from build123d import *

# Parameters (mm, degrees)
F2_T     = 3.175
F3_R     = 6.35
F4_DEPTH = 64.008
F5_DEPTH = 104.14


# Not quite as in the source:
# - a shell that OpenCascade refuses in one call is made with other operations: the cavity is built on its own and cut out


with BuildPart() as f1:
    # F0 (on Top) → F1 (revolve)
    with BuildSketch(Plane.XY):
        Polygon((-37.0614958425, 0), (0, 0), (0, 59.2983933481), (-37.0614958425, 59.2983933481), (-37.0614958425, 54.4952234869), (-29.1296224819, 54.4952234869), (-29.1296224819, 50.8915618087), (-37.0614958425, 50.8915618087), (-37.0614958425, 46.1002111902), (-29.1296224819, 46.1002111902), (-29.1296224819, 42.483009196), (-37.0614958425, 42.483009196), (-37.0614958425, 37.6798393348), (-29.1296224819, 37.6798393348), (-29.1296224819, 31.75), (-37.0614958425, 31.75), align=None)
    revolve(axis=Axis((0, 29.649196674, 0), (0, 1, 0)))

    # F2: shell of thickness 3.175, made by hand


with BuildPart() as f2_core1:
    # F2_t2: copy of F1
    add(f1.part)

    # the walls: a layer under each face that stays
    f2_faces = [f2_core1.faces().sort_by_distance(p)[0] for p in [
        (29.1296224819, 34.7149196674, 0),
        (-24.707663895, 31.75, -24.707663895),
        (37.0614958425, 15.875, 0),
        (0, 59.2983933481, 0),
        (37.0614958425, 56.8968084175, 0),
        (24.707663895, 54.4952234869, -24.707663895),
        (29.1296224819, 52.6933926478, 0),
        (-24.707663895, 50.8915618087, -24.707663895),
        (37.0614958425, 48.4958864995, 0),
        (24.707663895, 46.1002111902, -24.707663895),
        (29.1296224819, 44.2916101931, 0),
        (-24.707663895, 42.483009196, -24.707663895),
        (37.0614958425, 40.0814242654, 0),
        (24.707663895, 37.6798393348, -24.707663895),
    ]]
    thicken(f2_faces, amount=-F2_T, mode=Mode.SUBTRACT)

    # F2_s3 → F2_t4 (revolve, cut)
    with BuildSketch(Plane.XY):
        Polygon((-29.1613724819, 37.6480893348), (-25.9546224819, 37.6798393348), (-25.9546224819, 40.8548393348), (-29.1296224819, 40.8548393348), align=None)
    revolve(axis=Axis((0, 37.6798393348, 0), (0, 1, 0)), mode=Mode.SUBTRACT)

    # F2_s5 → F2_t6 (revolve, cut)
    with BuildSketch(Plane.XY):
        Polygon((-29.1613724819, 31.78175), (-25.9546224819, 31.75), (-25.9546224819, 28.575), (-29.1296224819, 28.575), align=None)
    revolve(axis=Axis((0, 31.75, 0), (0, 1, 0)), mode=Mode.SUBTRACT)

    # F2_s7 → F2_t8 (revolve, cut)
    with BuildSketch(Plane.XY):
        Polygon((-29.1613724819, 54.4634734869), (-29.1296224819, 57.6702234869), (-25.9546224819, 57.6702234869), (-25.9546224819, 54.4952234869), align=None)
    revolve(axis=Axis((0, 54.4952234869, 0), (0, 1, 0)), mode=Mode.SUBTRACT)

    # F2_s9 → F2_t10 (revolve, cut)
    with BuildSketch(Plane.XY):
        Polygon((-29.1613724819, 50.9233118087), (-25.9546224819, 50.8915618087), (-25.9546224819, 47.7165618087), (-29.1296224819, 47.7165618087), align=None)
    revolve(axis=Axis((0, 50.8915618087, 0), (0, 1, 0)), mode=Mode.SUBTRACT)

    # F2_s11 → F2_t12 (revolve, cut)
    with BuildSketch(Plane.XY):
        Polygon((-29.1613724819, 46.0684611902), (-29.1296224819, 49.2752111902), (-25.9546224819, 49.2752111902), (-25.9546224819, 46.1002111902), align=None)
    revolve(axis=Axis((0, 46.1002111902, 0), (0, 1, 0)), mode=Mode.SUBTRACT)

    # F2_s13 → F2_t14 (revolve, cut)
    with BuildSketch(Plane.XY):
        Polygon((-29.1613724819, 42.514759196), (-25.9546224819, 42.483009196), (-25.9546224819, 39.308009196), (-29.1296224819, 39.308009196), align=None)
    revolve(axis=Axis((0, 42.483009196, 0), (0, 1, 0)), mode=Mode.SUBTRACT)


with BuildPart() as f1_1:
    add(f1.part)

    # what is left inside the walls is the cavity
    f2_cavity = [f2_core1.part.solids().sort_by_distance(p)[0] for p in [
        (33.854746, 19.05, 0),
    ]]
    add(f2_cavity, mode=Mode.SUBTRACT)

    # F3 (on Top) → F4 (cut)
    with BuildSketch(Plane.XY):
        with Locations((0, 20.6699799746)):
            Circle(F3_R)
    extrude(amount=-F4_DEPTH, mode=Mode.SUBTRACT)

    # F3 (on Top) → F5 (cut)
    with BuildSketch(Plane.XY):
        with Locations((0, 20.6699799746)):
            Circle(F3_R)
    extrude(amount=F5_DEPTH, mode=Mode.SUBTRACT)


solid = f1_1.part
For this review, take the finished solid that the model builds, in its own axes (mm). A direction names the side the tool comes from. Round coordinates to 2 decimals unless told otherwise and drop trailing zeros. Order: outer loops, then holes, each group sorted by start corner. A loop starts at its lowest first (then second) coordinate and runs counter-clockwise, first axis right, second up. Notation, with made-up numbers: (34, 55.25) -> (75, 55.25) arc R19 ccw to (75, 61.25) -> close; hole circle Ø4 at (35.5, 81). An arc over 180 degrees is marked (long way). Put each result on its own line as item: value.
Q1. Mouldability with a two-part tool opening along Y and no side actions: class faces 4 (the cylindrical face through (4.825, 48.462, 36.746)), 5 (the flat face through (16, 50.892, -25)), 6 (the flat face through (-8, 28.575, -25)), 7 (the flat face through (-16, 46.1, -25)) as pulls with the +Y half, pulls with the -Y half, needs draft (parallel to the pull), parting line crosses it, or undercut.
Check result:
face 4: needs draft
face 5: undercut
face 6: pulls with the -Y half
face 7: undercut
Q2. Add section A-A on x = 0. State how many separate pieces and enclosed holes the cut face has, plus the area to 3 significant figures.
Check result:
separate pieces: 3
enclosed holes: 0
area: 739 mm2
Q3. Insertion check: pin 1 Ø1.5 at (x, y) = (13.5, 34) entering from +Z; pin 2 Ø5 at (y, z) = (10.5, -29) entering from -X; pin 3 Ø11.5 at (x, y) = (0, 20.67) entering from -Z; pin 4 Ø12 at (x, z) = (5, 5) entering from -Y. Each pin has a flat end and moves straight along its axis. Give the tip position at first contact, or say it passes through.
Check result:
pin 1: z = 26.19
pin 2: x = -25.91
pin 3: through
pin 4: y = 56.12
Q4. Add section B-B on y = 53. Write out the cut boundary in (x, z), plus the area to 3 significant figures.
Check result:
outline: circle Ø58.26 at (0, 0); hole circle Ø51.91 at (0, 0)
area: 549 mm2
Q5. Machinability: for faces 1 (the cylindrical face through (6.31, 52.67, -28.44)), 2 (the flat face through (-16.3, 0, -30)), 3 (the cylindrical face through (5.626, 42.156, -25.337)), which of the approach directions +Z, -Z, +X, -X, +Y, -Y give a long, thin tool a straight path to every point of the face, cutting with its end or side? Answer none if there is none.
Check result:
face 1: none
face 2: +Z, -Z, +X, -X, -Y
face 3: -Y
Q6. For probe 1 along Y at (x, z) = (0, -34.1); probe 2 along Y at (x, z) = (8.5, 29.5) (3 decimals); probe 3 along Z at (x, y) = (0, 37.5), list the stretches that pass through material, from the lowest coordinate up. Write a range as [from, to].
Check result:
probe 1: [0, 14.32], [27.02, 31.75], [37.68, 42.48], [46.1, 50.89], [54.5, 59.3]
probe 2: [28.575, 31.75], [37.68, 42.483], [46.1, 50.892], [54.495, 59.298]
probe 3: [-29.13, -25.95], [25.95, 29.13]
